Geometry check sheet. Reference: the model listing, model coordinates, mm. A direction names the side the tool comes from. Coordinates: 2 decimals unless noted, no trailing zeros. Write each loop counter-clockwise with the first axis right and the second up, starting at its lowest first coordinate (ties: lowest second). Pieces come first, ordered by that corner, then holes. Notation, with made-up numbers: M -37.75,-19 L 5.25,-19 A21 cw 5.25,1 Z; hole C 55,85 d8. An arc over 180 degrees is marked long. Answer as a JSON object with one key per item and string values. Group by question number.
Autodesk Inventor part; units mm, degrees
ref_plane "YZ Plane" through (0, 0, 0) normal (1, 0, 0) x (0, 1, 0)
ref_plane "XZ Plane" through (0, 0, 0) normal (0, 1, 0) x (-1, 0, 0)
ref_plane "XY Plane" through (0, 0, 0) normal (0, 0, 1) x (1, 0, 0)
sketch "Sketch1" plane through (0, 0, 0) normal (0, 1, 0) x (-1, 0, 0)
  line L0 (0, -2.6558) -> (-2.3, -1.3279)
  line L1 (-2.3, -1.3279) -> (-2.3, 1.3279)
  line L2 (-2.3, 1.3279) -> (0, 2.6558)
  line L3 (0, 2.6558) -> (2.3, 1.3279)
  line L4 (2.3, 1.3279) -> (2.3, -1.3279)
  line L5 (2.3, -1.3279) -> (0, -2.6558)
  circle A0 centre (0, 0) radius 1.45
  dimension "d4" = 2.9
  dimension "d5" = 4.6
extrude "Extrusion1" add sketch "Sketch1" along normal blind 12 contours L0 L1 L2 L3 L4 L5 | A0
extrude "Extrusion2" add sketch "Sketch1" against normal blind 5 contours A0
sketch "Sketch2" plane through (0, 12, 0) normal (0, 1, 0) x (1, 0, 0)
  circle A0 centre (0, 0) radius 1.45
  circle A1 centre (0, 0) radius 1.45
  circle A2 centre (0, 0) radius 1.5
  dimension "d6" = 3
extrude "Extrusion3" cut sketch "Sketch2" against normal blind 10 contours A0 | A2
properties part number "mounting"
1) Material ranges on probe 1 along X at (y, z) = (9.75, 0); probe 2 along Y at (x, z) = (-0.35, 1.35); probe 3 along Y at (x, z) = (-1.3, -1.55), recorded low to high. Write a range as [from, to].
2) Draft check along Z on faces 4 (the cylindrical face through (1.45, -2.46, 0.06)), 5 (the flat face through (0, 2, 0)), 6 (the flat face through (1.17, 5.92, 1.98)), 7 (the flat face through (2, 12, 0)). Enter one of: +Z half, -Z half, draft (parallel to the pull), parting line (faces both ways), or undercut.
3) Section check D-D (y = -2.5). Record the cut outline in (x, z), then the cut area to 3 significant figures.
4) Section check A-A (y = 4). Record the cut outline in (x, z).
5) Section check B-B (z = 0). Record the cut outline in (x, y).
6) Go/stop test with flat-tipped pins: pin 1 Ø2 at (y, z) = (-2.5, -1) entering from +X; pin 2 Ø1.5 at (x, y) = (-1.5, 7) entering from -Z. Record where each tip stops, or that it passes through.
7) Section check C-C (x = 0.4). Record the cut outline in (y, z), then the cut area to 3 significant figures.
8) Set-up check for faces 1 (the cylindrical face through (-1.5, 7.07, -0.07)), 2 (the flat face through (-1.17, 5.92, -1.98)), 3 (the flat face through (2, 0, 0)): record each of +Z, -Z, +X, -X, +Y, -Y from which the full face is reachable in a straight line by a thin tool's end or side.
Entries:
{
 "1": {"probe 1": "[-2.3, -1.5], [1.5, 2.3]", "probe 2": "[-5, 2]", "probe 3": "[0, 12]"},
 "2": {"face 4": "parting line", "face 5": "undercut", "face 6": "+Z half", "face 7": "draft"},
 "3": {"outline": "C 0,0 d2.9", "area": "6.61 mm^2"},
 "4": {"outline": "M -2.3,-1.33 L 0,-2.66 L 2.3,-1.33 L 2.3,1.33 L 0,2.66 L -2.3,1.33 Z; hole C 0,0 d3"},
 "5": {"outline": "M -2.3,0 L -1.45,0 L -1.45,-5 L 1.45,-5 L 1.45,0 L 2.3,0 L 2.3,12 L 1.5,12 L 1.5,2 L -1.5,2 L -1.5,12 L -2.3,12 Z"},
 "6": {"pin 1": "x = 1.45", "pin 2": "z = -2.22"},
 "7": {"outline": "M -5,-1.39 L 0,-1.39 L 0,-2.42 L 12,-2.42 L 12,-1.45 L 2,-1.45 L 2,1.45 L 12,1.45 L 12,2.42 L 0,2.42 L 0,1.39 L -5,1.39 Z", "area": "43.2 mm^2"},
 "8": {"face 1": "+Y", "face 2": "-Z, -X, +Y, -Y", "face 3": "-Y"}
}
